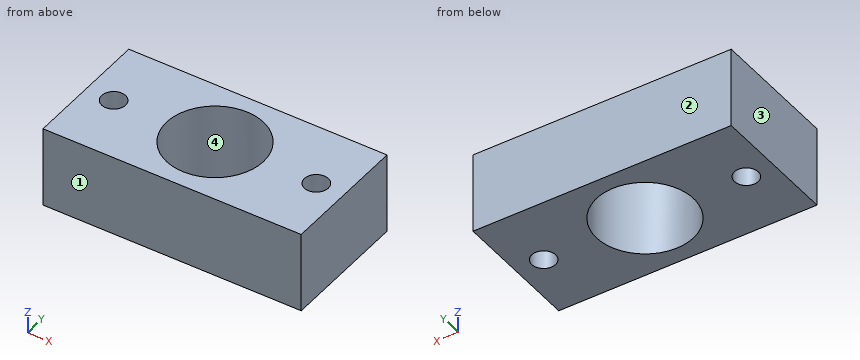
from build123d import *

# Parameters (mm, degrees)
F0_W     = 101.6
F0_H     = 50.8
F1_DEPTH = 31.75
F2_R     = 19.05
F3_DEPTH = 31.751
F4_R     = 4.699
F5_DEPTH = 31.751


with BuildPart() as f1:
    # F0 (on Top) → F1 (new body)
    with BuildSketch(Plane.XY):
        Rectangle(F0_W, F0_H)
    extrude(amount=F1_DEPTH)

    # F2 (on Top) → F3 (cut, through all)
    with BuildSketch(Plane.XY):
        Circle(F2_R)
    extrude(amount=F3_DEPTH, mode=Mode.SUBTRACT)

    # F4 (on Top) → F5 (cut, through all)
    with BuildSketch(Plane.XY):
        with Locations((-39.878, 0)):
            Circle(F4_R)
        with Locations((39.878, 0)):
            Circle(F4_R)
    extrude(amount=F5_DEPTH, mode=Mode.SUBTRACT)


solid = f1.part
CAD build for the part. Positions are in the model's coordinates, mm. Face numbers are marked on the shaded views. Round coordinates to 2 decimals unless told otherwise and drop trailing zeros. Write each loop counter-clockwise with the first axis right and the second up, starting at its lowest first coordinate (ties: lowest second). Pieces come first, ordered by that corner, then holes.
(1) Probe line 1 along X through (y, z) = (0, 15); line 2 along Y through (x, z) = (0, 24); line 3 along X through (y, z) = (-15, 4.5). List the from-to ranges inside material, lowest first.
(2) Slice it at C-C, the plane x = 0. Write the cut outline in (y, z), and give its area (3 significant figures).
(3) Slice it at B-B, the plane y = 0. Write the cut outline in (x, z), and give its area (3 significant figures).
(4) Mould opens along Y. For the marked faces 1, 2, 3 and 4 say: pulls with the +Y half, pulls with the -Y half, needs draft (parallel to the pull), parting line crosses it, or undercut.
(5) Slice it at A-A, the plane z = 21.5. Write the cut outline in (x, y).
(6) Drop a flat-ended pin along its axis: P1, Ø15, axis at x = 39.878, y = 0, coming from the -Z side. Give the stop position or say it passes through.
(7) Slice it at D-D, the plane y = -11. Write the cut outline in (x, z).
From the geometry:
1. line 1: x = -50.8 to -44.58, -35.18 to -19.05, 19.05 to 35.18, 44.58 to 50.8
1. line 2: y = -25.4 to -19.05, 19.05 to 25.4
1. line 3: x = -50.8 to -11.74, 11.74 to 50.8
2. outline: (-25.4, 0) - (-19.05, 0) - (-19.05, 31.75) - (-25.4, 31.75) - close; (19.05, 0) - (25.4, 0) - (25.4, 31.75) - (19.05, 31.75) - close
2. area: 403 mm2
3. outline: (-50.8, 0) - (-44.58, 0) - (-44.58, 31.75) - (-50.8, 31.75) - close; (-35.18, 0) - (-19.05, 0) - (-19.05, 31.75) - (-35.18, 31.75) - close; (19.05, 0) - (35.18, 0) - (35.18, 31.75) - (19.05, 31.75) - close; (44.58, 0) - (50.8, 0) - (50.8, 31.75) - (44.58, 31.75) - close
3. area: 1,420 mm2
4. face 1: pulls with the -Y half
4. face 2: pulls with the +Y half
4. face 3: needs draft
4. face 4: undercut
5. outline: (-50.8, -25.4) - (50.8, -25.4) - (50.8, 25.4) - (-50.8, 25.4) - close; hole circle Ø9.4 at (-39.88, 0); hole circle Ø38.1 at (0, 0); hole circle Ø9.4 at (39.88, 0)
6. P1: stops at z = 0
7. outline: (-50.8, 0) - (-15.55, 0) - (-15.55, 31.75) - (-50.8, 31.75) - close; (15.55, 0) - (50.8, 0) - (50.8, 31.75) - (15.55, 31.75) - close
